Check sheet for the modelled part. Datum: model origin and axes. Units: mm. A direction names the side the tool comes from. Round coordinates to 2 decimals unless told otherwise and drop trailing zeros. Write each loop counter-clockwise with the first axis right and the second up, starting at its lowest first coordinate (ties: lowest second). Pieces come first, ordered by that corner, then holes.
Item 1: Material ranges on line 1 along Z through (x, y) = (269, 289.5); line 2 along X through (y, z) = (295.75, -6.5); line 3 along Y through (x, z) = (294.5, -71), recorded low to high.
Item 2: Section check A-A, the plane z = -41.5. Record the cut outline in (x, y), plus the area to 3 significant figures.
Item 3: Depth check by flat-ended pin: pin 1 (1.8 mm diameter, centred on x = 294, y = 296.5, fed in from -Z); pin 2 (3 mm diameter, centred on y = 300, z = -28.5, fed in from +X); pin 3 (0.8 mm diameter, centred on x = 294.5, y = 305.5, fed in from -Z). Enter the tip coordinate at first touch or a pass-through.
Item 4: Set-up check for faces 1 (the flat face through (251, 282, -23)), 2 (the flat face through (273, 282.5, -83)), 3 (the flat face through (273, 306, -49)), 4 (the flat face through (273, 293, -50)): record each of +Z, -Z, +X, -X, +Y, -Y from which the full face is reachable in a straight line by a thin tool's end or side.
Item 5: Section check B-B, the plane y = 302.25. Record the cut outline in (x, z).
Item 6: Section check C-C, the plane z = -62. Record the cut outline in (x, y).
Item 7: Release check for a two-part mould opening along Z. For faces 5 (the flat face through (275, 293, 2.5)), 6 (the cylindrical face through (262.75, 281.23, -103.62)), 7 (the flat face through (296.5, 293, -25)) record: pulls with the +Z half, pulls with the -Z half, needs draft (parallel to the pull), parting line crosses it, or undercut.
from build123d import *

# Parameters (mm, degrees)
BASE_FLANGE1_OUTLINE_W       = 50
BASE_FLANGE1_OUTLINE_H       = 62.620541263
BASE_FLANGE1_OUTLINE_R       = 1.849849123
BASE_FLANGE1_DEPTH           = 2.5
EDGE_FLANGE1_STRIP_W         = 12
EDGE_FLANGE1_STRIP_H         = 2.5
EDGE_FLANGE1_STRIP_CUT_DEPTH = 62.620541263
EDGE_FLANGE1_DEPTH           = 62.620541263
EDGE_FLANGE2_STRIP_W         = 12
EDGE_FLANGE2_STRIP_H         = 2.5
EDGE_FLANGE2_STRIP_CUT_DEPTH = 46.5
EDGE_FLANGE2_DEPTH           = 46.5
EDGE_FLANGE4_STRIP_W         = 12
EDGE_FLANGE4_STRIP_H         = 2.5
EDGE_FLANGE4_STRIP_CUT_DEPTH = 46.5
EDGE_FLANGE4_DEPTH           = 46.5
EDGE_FLANGE5_STRIP_W         = 12
EDGE_FLANGE5_STRIP_H         = 2.5
EDGE_FLANGE5_STRIP_CUT_DEPTH = 51.5
EDGE_FLANGE5_DEPTH           = 51.5
EDGE_FLANGE6_STRIP_W         = 12
EDGE_FLANGE6_STRIP_H         = 2.5
EDGE_FLANGE6_STRIP_CUT_DEPTH = 43
EDGE_FLANGE6_DEPTH           = 43
EDGE_FLANGE7_STRIP_W         = 12
EDGE_FLANGE7_STRIP_H         = 2.5
EDGE_FLANGE7_STRIP_CUT_DEPTH = 48
EDGE_FLANGE7_DEPTH           = 48
SKETCH31_W                   = 39.5
SKETCH31_H                   = 48
CUT_EXTRUDE1_DEPTH           = 4


# Read off the part's stored shape, not the designer's step: Base-Flange1
# Sheet-metal steps are written as plain solids
with BuildPart() as part:
    # Base-Flange1 outline → Base-Flange1 (new body)
    with BuildSketch(Plane(origin=(0, 280, 0), x_dir=(1, 0, 0), z_dir=(0, 1, 0))):
        with Locations((275, 81.310270632)):
            Rectangle(BASE_FLANGE1_OUTLINE_W, BASE_FLANGE1_OUTLINE_H)
        with Locations((264.597334147, 103.542995429)):
            Circle(BASE_FLANGE1_OUTLINE_R, mode=Mode.SUBTRACT)
        with Locations((285.402665853, 103.542995429)):
            Circle(BASE_FLANGE1_OUTLINE_R, mode=Mode.SUBTRACT)
    extrude(amount=BASE_FLANGE1_DEPTH)

    # Edge-Flange1 strip (across the edge) → Edge-Flange1 strip cut (cut)
    with BuildSketch(Plane(origin=(300, 282.5, -50), x_dir=(-1, 0, 0), z_dir=(0, 0, -1))):
        with Locations((-2.5, -1.25)):
            Rectangle(EDGE_FLANGE1_STRIP_W, EDGE_FLANGE1_STRIP_H)
    extrude(amount=EDGE_FLANGE1_STRIP_CUT_DEPTH, mode=Mode.SUBTRACT)

    # Edge-Flange1 section (across the edge) → Edge-Flange1 (add)
    with BuildSketch(Plane(origin=(300, 282.5, -50), x_dir=(-1, 0, 0), z_dir=(0, 0, -1))):
        with BuildLine():
            Line((0, 1), (0, 26.2366))
            Line((0, 26.2366), (2.5, 26.2366))
            Line((2.5, 26.2366), (2.5, 1))
            ThreePointArc((2.5, 1), (2.792893219, 0.292893219), (3.5, 0))
            Line((3.5, 0), (3.5, -2.5))
            ThreePointArc((3.5, -2.5), (1.025126266, -1.474873734), (0, 1))
        make_face()
    extrude(amount=EDGE_FLANGE1_DEPTH)

    # Edge-Flange2 strip (across the edge) → Edge-Flange2 strip cut (cut)
    with BuildSketch(Plane(origin=(250, 282.5, -50), x_dir=(0, 0, -1), z_dir=(1, 0, 0))):
        with Locations((-2.5, -1.25)):
            Rectangle(EDGE_FLANGE2_STRIP_W, EDGE_FLANGE2_STRIP_H)
    extrude(amount=EDGE_FLANGE2_STRIP_CUT_DEPTH, mode=Mode.SUBTRACT)

    # Edge-Flange2 section (across the edge) → Edge-Flange2 (add)
    with BuildSketch(Plane(origin=(250, 282.5, -50), x_dir=(0, 0, -1), z_dir=(1, 0, 0))):
        with BuildLine():
            Line((0, 1), (0, 24.5))
            Line((0, 24.5), (2.5, 24.5))
            Line((2.5, 24.5), (2.5, 1))
            ThreePointArc((2.5, 1), (2.792893219, 0.292893219), (3.5, 0))
            Line((3.5, 0), (3.5, -2.5))
            ThreePointArc((3.5, -2.5), (1.025126266, -1.474873734), (0, 1))
        make_face()
    extrude(amount=EDGE_FLANGE2_DEPTH)

    # Edge-Flange4 strip (across the edge) → Edge-Flange4 strip cut (cut)
    with BuildSketch(Plane(origin=(296.5, 307, -50), x_dir=(0, -1, 0), z_dir=(-1, 0, 0))):
        with Locations((-2.5, -1.25)):
            Rectangle(EDGE_FLANGE4_STRIP_W, EDGE_FLANGE4_STRIP_H)
    extrude(amount=EDGE_FLANGE4_STRIP_CUT_DEPTH, mode=Mode.SUBTRACT)

    # Edge-Flange4 section (across the edge) → Edge-Flange4 (add)
    with BuildSketch(Plane(origin=(296.5, 307, -50), x_dir=(0, -1, 0), z_dir=(-1, 0, 0))):
        with BuildLine():
            Line((0, 1), (0, 52.5))
            Line((0, 52.5), (2.5, 52.5))
            Line((2.5, 52.5), (2.5, 1))
            ThreePointArc((2.5, 1), (2.792893219, 0.292893219), (3.5, 0))
            Line((3.5, 0), (3.5, -2.5))
            ThreePointArc((3.5, -2.5), (1.025126266, -1.474873734), (0, 1))
        make_face()
    extrude(amount=EDGE_FLANGE4_DEPTH)

    # Edge-Flange5 strip (across the edge) → Edge-Flange5 strip cut (cut)
    with BuildSketch(Plane(origin=(250, 304.5, 2.5), x_dir=(1, 0, 0), z_dir=(0, 0, -1))):
        with Locations((-2.5, -1.25)):
            Rectangle(EDGE_FLANGE5_STRIP_W, EDGE_FLANGE5_STRIP_H)
    extrude(amount=EDGE_FLANGE5_STRIP_CUT_DEPTH, mode=Mode.SUBTRACT)

    # Edge-Flange5 section (across the edge) → Edge-Flange5 (add)
    with BuildSketch(Plane(origin=(250, 304.5, 2.5), x_dir=(1, 0, 0), z_dir=(0, 0, -1))):
        with BuildLine():
            Line((0, 1), (0, 22.5))
            Line((0, 22.5), (2.5, 22.5))
            Line((2.5, 22.5), (2.5, 1))
            ThreePointArc((2.5, 1), (2.792893219, 0.292893219), (3.5, 0))
            Line((3.5, 0), (3.5, -2.5))
            ThreePointArc((3.5, -2.5), (1.025126266, -1.474873734), (0, 1))
        make_face()
    extrude(amount=EDGE_FLANGE5_DEPTH)

    # Edge-Flange6 strip (across the edge) → Edge-Flange6 strip cut (cut)
    with BuildSketch(Plane(origin=(296.5, 304.5, 2.5), x_dir=(0, 0, -1), z_dir=(-1, 0, 0))):
        with Locations((-2.5, -1.25)):
            Rectangle(EDGE_FLANGE6_STRIP_W, EDGE_FLANGE6_STRIP_H)
    extrude(amount=EDGE_FLANGE6_STRIP_CUT_DEPTH, mode=Mode.SUBTRACT)

    # Edge-Flange6 section (across the edge) → Edge-Flange6 (add)
    with BuildSketch(Plane(origin=(296.5, 304.5, 2.5), x_dir=(0, 0, -1), z_dir=(-1, 0, 0))):
        with BuildLine():
            Line((0, 1), (0, 22.5))
            Line((0, 22.5), (2.5, 22.5))
            Line((2.5, 22.5), (2.5, 1))
            ThreePointArc((2.5, 1), (2.792893219, 0.292893219), (3.5, 0))
            Line((3.5, 0), (3.5, -2.5))
            ThreePointArc((3.5, -2.5), (1.025126266, -1.474873734), (0, 1))
        make_face()
    extrude(amount=EDGE_FLANGE6_DEPTH)

    # Edge-Flange7 strip (across the edge) → Edge-Flange7 strip cut (cut)
    with BuildSketch(Plane(origin=(296.5, 304.5, -49), x_dir=(-1, 0, 0), z_dir=(0, 0, 1))):
        with Locations((-2.5, -1.25)):
            Rectangle(EDGE_FLANGE7_STRIP_W, EDGE_FLANGE7_STRIP_H)
    extrude(amount=EDGE_FLANGE7_STRIP_CUT_DEPTH, mode=Mode.SUBTRACT)

    # Edge-Flange7 section (across the edge) → Edge-Flange7 (add)
    with BuildSketch(Plane(origin=(296.5, 304.5, -49), x_dir=(-1, 0, 0), z_dir=(0, 0, 1))):
        with BuildLine():
            Line((0, 1), (0, 22.5))
            Line((0, 22.5), (2.5, 22.5))
            Line((2.5, 22.5), (2.5, 1))
            ThreePointArc((2.5, 1), (2.792893219, 0.292893219), (3.5, 0))
            Line((3.5, 0), (3.5, -2.5))
            ThreePointArc((3.5, -2.5), (1.025126266, -1.474873734), (0, 1))
        make_face()
    extrude(amount=EDGE_FLANGE7_DEPTH)

    # Sketch31 → Cut-Extrude1 (cut)
    with BuildSketch(Plane(origin=(0, 307, 0), x_dir=(1, 0, 0), z_dir=(0, 1, 0))):
        with Locations((273.25, 25)):
            Rectangle(SKETCH31_W, SKETCH31_H)
    extrude(amount=-CUT_EXTRUDE1_DEPTH, mode=Mode.SUBTRACT)


solid = part.part
Values found:
1. line 1: z = -52.5 to -50, 0 to 2.5
1. line 2: x = 250 to 252.5, 294 to 296.5
1. line 3: y = 280 to 282.5
2. outline: (250, 282) - (252.5, 282) - (252.5, 303.5) arc R1 cw to (253.5, 304.5) - (253.5, 307) arc R3.5 ccw to (250, 303.5) - close; (293, 304.5) arc R1 cw to (294, 303.5) - (294, 282) - (296.5, 282) - (296.5, 303.5) arc R3.5 ccw to (293, 307) - close
2. area: 125 mm2
3. pin 1: stops at z = -52.5
3. pin 2: stops at x = 296.5
3. pin 3: stops at z = -52.11
4. face 1: +Z, +X, -X, -Y
4. face 2: -Z, -X, +Y
4. face 3: +Y, -Y
4. face 4: +X, -X, -Y
5. outline: (250, -52.5) - (296.5, -52.5) - (296.5, -50) - (250, -50) - close; (250, -49) - (252.5, -49) - (252.5, 2.5) - (250, 2.5) - close; (253.5, 0) - (296.5, 0) - (296.5, 2.5) - (253.5, 2.5) - close; (294, -49) - (296.5, -49) - (296.5, -1) - (294, -1) - close; (297.5, -112.62) - (300, -112.62) - (300, -50) - (297.5, -50) - close
6. outline: (250, 280) - (296.5, 280) arc R3.5 ccw to (300, 283.5) - (300, 308.74) - (297.5, 308.74) - (297.5, 283.5) arc R1 cw to (296.5, 282.5) - (250, 282.5) - close
7. face 5: pulls with the +Z half
7. face 6: undercut
7. face 7: needs draft
